from build123d import *

# Parameters (mm, degrees)
SKETCH1_R               = 1.651
BOSS_EXTRUDE2_DEPTH     = 3.175
SKETCH3_R               = 12.1285
CUT_EXTRUDE2_DEPTH      = 4.175
SKETCH4_W               = 37.082318314
SKETCH4_H               = 34.047903563
SKETCH4_W_2             = 37.024578492
SKETCH4_H_2             = 32.488734362
BOSS_EXTRUDE3_DEPTH     = 3.175
SKETCH5_R               = 5
CUT_EXTRUDE3_DEPTH      = 4.175
SKETCH6_R               = 3.175
CUT_EXTRUDE4_DEPTH      = 1
CUT_EXTRUDE4_DEPTH_BACK = 4.175
SKETCH7_R               = 1.651
CUT_EXTRUDE5_DEPTH      = 16.51


with BuildPart() as part:
    # Sketch1 → Boss-Extrude2 (new body)
    with BuildSketch(Plane.XY):
        with BuildLine():
            Line((-66.623575407, 34.29), (-54.685575407, 34.29))
            Line((-54.685575407, 34.29), (-54.685575407, -34.29))
            Line((-54.685575407, -34.29), (-66.623575407, -34.29))
            ThreePointArc((-66.623575407, -34.29), (0, -74.93), (66.623575407, -34.29))
            Line((66.623575407, -34.29), (54.685575407, -34.29))
            Line((54.685575407, -34.29), (54.685575407, 34.29))
            Line((54.685575407, 34.29), (66.623575407, 34.29))
            ThreePointArc((66.623575407, 34.29), (0, 74.93), (-66.623575407, 34.29))
        make_face()
        with Locations((-45.466, 11.049)):
            Circle(SKETCH1_R, mode=Mode.SUBTRACT)
        with Locations((-20.067270032, 10.795)):
            Circle(SKETCH1_R, mode=Mode.SUBTRACT)
        with Locations((-20.067270032, -10.795)):
            Circle(SKETCH1_R, mode=Mode.SUBTRACT)
        with Locations((-45.466, -11.049)):
            Circle(SKETCH1_R, mode=Mode.SUBTRACT)
        with Locations((45.466, -11.049)):
            Circle(SKETCH1_R, mode=Mode.SUBTRACT)
        with Locations((20.067270032, -10.795)):
            Circle(SKETCH1_R, mode=Mode.SUBTRACT)
        with Locations((20.067270032, 10.795)):
            Circle(SKETCH1_R, mode=Mode.SUBTRACT)
        with Locations((45.466, 11.049)):
            Circle(SKETCH1_R, mode=Mode.SUBTRACT)
    extrude(amount=BOSS_EXTRUDE2_DEPTH)

    # Sketch3 → Cut-Extrude2 (cut, through all)
    with BuildSketch(Plane(origin=(0, 0, 0), x_dir=(-1, 0, 0), z_dir=(0, 0, -1))):
        with Locations((0, -13.208)):
            Circle(SKETCH3_R)
        with Locations((0, 13.208)):
            Circle(SKETCH3_R)
        with Locations((-43.105229381, -43.105229381)):
            Circle(SKETCH3_R)
        with Locations((19.05, -32.995567884)):
            Circle(SKETCH3_R)
        with Locations((19.05, 32.995567884)):
            Circle(SKETCH3_R)
        with Locations((-43.105229381, 43.105229381)):
            Circle(SKETCH3_R)
        with Locations((43.105229381, 43.105229381)):
            Circle(SKETCH3_R)
        with Locations((-19.05, 32.995567884)):
            Circle(SKETCH3_R)
        with Locations((-19.05, -32.995567884)):
            Circle(SKETCH3_R)
        with Locations((43.105229381, -43.105229381)):
            Circle(SKETCH3_R)
    extrude(amount=-CUT_EXTRUDE2_DEPTH, mode=Mode.SUBTRACT)

    # Sketch4 → Boss-Extrude3 (add)
    with BuildSketch(Plane(origin=(0, 0, 0), x_dir=(-1, 0, 0), z_dir=(0, 0, -1))):
        with Locations((32.991199211, -1.421154886)):
            Rectangle(SKETCH4_W, SKETCH4_H)
        with Locations((-34.085074962, -0.641570285)):
            Rectangle(SKETCH4_W_2, SKETCH4_H_2)
    extrude(amount=-BOSS_EXTRUDE3_DEPTH)

    # Sketch5 → Cut-Extrude3 (cut, through all)
    with BuildSketch(Plane(origin=(0, 0, 0), x_dir=(-1, 0, 0), z_dir=(0, 0, -1))):
        with Locations((34.29, -15.24)):
            Circle(SKETCH5_R)
        with Locations((-34.29, -15.24)):
            Circle(SKETCH5_R)
        with Locations((34.29, 15.24)):
            Circle(SKETCH5_R)
        with Locations((-34.29, 15.24)):
            Circle(SKETCH5_R)
    extrude(amount=-CUT_EXTRUDE3_DEPTH, mode=Mode.SUBTRACT)

    # Sketch6 → Cut-Extrude4 (cut, two sides)
    with BuildSketch(Plane(origin=(31.313436391, -132.613959999, 3.175), x_dir=(0, -1, 0), z_dir=(0, 0, 1))) as cut_extrude4_sk:
        with Locations((-158.013959999, 14.406563609)):
            Circle(SKETCH6_R)
        with Locations((-169.443959999, -31.313436391)):
            Circle(SKETCH6_R)
        with Locations((-158.013959999, -77.033436391)):
            Circle(SKETCH6_R)
        with Locations((-107.213959999, -77.033436391)):
            Circle(SKETCH6_R)
        with Locations((-95.783959999, -31.313436391)):
            Circle(SKETCH6_R)
        with Locations((-107.213959999, 14.406563609)):
            Circle(SKETCH6_R)
    extrude(amount=CUT_EXTRUDE4_DEPTH, mode=Mode.SUBTRACT)
    extrude(cut_extrude4_sk.sketch, amount=-CUT_EXTRUDE4_DEPTH_BACK, mode=Mode.SUBTRACT)

    # Sketch7 → Cut-Extrude5 (cut)
    with BuildSketch(Plane(origin=(31.313436391, -132.613959999, 15.875), x_dir=(0, -1, 0), z_dir=(0, 0, 1))):
        with Locations((-198.653959999, -31.313436391)):
            Circle(SKETCH7_R)
        with Locations((-66.573959999, -31.313436391)):
            Circle(SKETCH7_R)
        with Locations((-132.613959999, -82.113436391)):
            Circle(SKETCH7_R)
        with Locations((-132.613959999, 19.486563609)):
            Circle(SKETCH7_R)
    extrude(amount=-CUT_EXTRUDE5_DEPTH, mode=Mode.SUBTRACT)


solid = part.part
Design review of the part built by this model. Coordinates are the model's own, in mm. A direction names the side the tool comes from. Give positions to 0.01 mm unless a question says otherwise; leave off trailing zeros. Write each loop counter-clockwise with the first axis right and the second up, starting at its lowest first coordinate (ties: lowest second). Pieces come first, ordered by that corner, then holes. Notation, with made-up numbers: M 63.25,83.5 L 116.25,83.5 A20 cw 116.25,118.5 Z; hole C 9,-5.5 d6. An arc over 180 degrees is marked long. Answer as a JSON object with one key per item and string values. Group by question number.
1) We need section C-C (x = -45.72). Give the boundary of the cut face in (y, z) (3 decimals).
2) We need section D-D (y = -4). Give the boundary of the cut face in (x, z) (3 decimals).
3) Tool access review of faces 4 (the face through (-52.4, 0.4, 1.6)), 5 (the face through (61, -34.29, 2)): name each direction out of +Z, -Z, +X, -X, +Y, -Y from which nothing blocks a thin tool from reaching the whole face with its end or side.
4) Mouldability with a two-part tool opening along X and no side actions: class faces 1 (the face through (-24.647, -43.756, 1.565)), 2 (the face through (-54.686, 0, 2)), 3 (the face through (-61, -34.29, 2)) as released by +X, released by -X, zero draft, split by the parting line, or undercut.
5) We need section B-B (x = 27.5). Give the boundary of the cut face in (y, z) (3 decimals).
6) Clearance check with flat-ended pins moving along their axes: pin 1 Ø4 at (x, y) = (-28.5, 16.5) entering from -Z; pin 2 Ø1 at (x, z) = (-3, 0.5) entering from +Y; pin 3 Ø1.5 at (x, z) = (-1, 1.5) entering from -Y; pin 4 Ø1 at (y, z) = (7.5, 2.5) entering from +X. State where each tip first meets the part, or that it passes through.
7) For line 1 along X through (y, z) = (0, 0.75); line 2 along X through (y, z) = (-48.5, 1.2); line 3 along X through (y, z) = (-40.5, 2), list the stretches that pass through material, from the lowest coordinate up.
8) We need section A-A (y = -36.83). Give the boundary of the cut face in (x, z) (3 decimals), and give its area (3 significant figures).
Answer key:
{
 "1": {"outline": "M -59.365,0 L -54.949,0 L -54.949,3.175 L -59.365,3.175 Z; M -31.262,0 L -28.575,0 L -28.575,3.175 L -31.262,3.175 Z; M -22.225,0 L 22.225,0 L 22.225,3.175 L -22.225,3.175 Z; M 28.575,0 L 31.262,0 L 31.262,3.175 L 28.575,3.175 Z; M 54.949,0 L 59.365,0 L 59.365,3.175 L 54.949,3.175 Z"},
 "2": {"outline": "M -54.686,0 L -7.894,0 L -7.894,3.175 L -54.686,3.175 Z; M 7.894,0 L 54.686,0 L 54.686,3.175 L 7.894,3.175 Z"},
 "3": {"face 4": "+Z, -Z", "face 5": "+Z, -Z, +X"},
 "4": {"face 1": "undercut", "face 2": "released by -X", "face 3": "zero draft"},
 "5": {"outline": "M -69.701,0 L -41.696,0 L -41.696,3.175 L -69.701,3.175 Z; M -24.295,0 L 24.295,0 L 24.295,3.175 L -24.295,3.175 Z; M 41.696,0 L 69.701,0 L 69.701,3.175 L 41.696,3.175 Z"},
 "6": {"pin 1": "stops at z = 0", "pin 2": "stops at y = 74.89", "pin 3": "stops at y = -74.93", "pin 4": "stops at x = 54.69"},
 "7": {"line 1": "x = -54.69 to -52.45, -49.15 to 49.15, 52.45 to 54.69", "line 2": "x = -57.12 to -53.97, -32.24 to 32.24, 53.97 to 57.12", "line 3": "x = -63.04 to -54.95, -31.26 to -28.58, -9.52 to 9.52, 28.58 to 31.26, 54.95 to 63.04"},
 "8": {"outline": "M -65.254,0 L -53.484,0 L -53.484,3.175 L -65.254,3.175 Z; M -32.726,0 L -30.556,0 L -30.556,3.175 L -32.726,3.175 Z; M -7.544,0 L -3.175,0 L -3.175,3.175 L -7.544,3.175 Z; M 3.175,0 L 7.544,0 L 7.544,3.175 L 3.175,3.175 Z; M 30.556,0 L 32.726,0 L 32.726,3.175 L 30.556,3.175 Z; M 53.484,0 L 65.254,0 L 65.254,3.175 L 53.484,3.175 Z", "area": "116 mm²"}
}
